from build123d import *

# Parameters (mm, degrees)
SKETCH001_W  = 7
SKETCH001_H  = 7
PAD001_DEPTH = 2
SKETCH_R     = 2.5
PAD_DEPTH    = 100


with BuildPart() as pad001:
    # Sketch001 → Pad001 (new body)
    with BuildSketch(Plane.YZ.offset(2)):
        with Locations((0, 59.5)):
            Rectangle(SKETCH001_W, SKETCH001_H)
    extrude(amount=PAD001_DEPTH)


with BuildPart() as cut:
    # Sketch → Pad (new body)
    with BuildSketch(Plane.XY):
        Circle(SKETCH_R)
    extrude(amount=PAD_DEPTH)

    # Cut: cut Pad001
    add(pad001.part, mode=Mode.SUBTRACT)


solid = cut.part
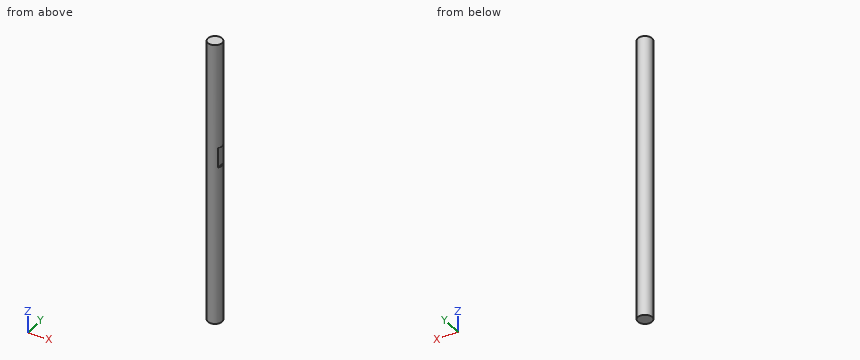
The model under review builds one solid part; all positions refer to its coordinate system, in mm. Coordinates: 2 decimals unless noted, no trailing zeros. Order: outer loops, then holes, each group sorted by start corner. A loop starts at its lowest first (then second) coordinate and runs counter-clockwise, first axis right, second up. Notation, with made-up numbers: (14.5, -13.75) -> (62.5, -13.75) arc R15 cw to (62.5, 3.25) -> close; hole circle Ø11 at (71, 89.5). An arc over 180 degrees is marked (long way). Answer in a Markdown table with one row per item.
(1) Consider section B-B (x = -1.5). Write out the cut boundary in (y, z), plus the area to 3 significant figures.
Answers:
| item | result |
|---|---|
| outline | (-2, 0) -> (2, 0) -> (2, 100) -> (-2, 100) -> close |
| area | 400 mm² |
(2) Insertion check: pin 1 (2 mm diameter, centred on y = 1, z = 60, fed in from -X); pin 2 (0.9 mm diameter, centred on y = -0.5, z = 58.5, fed in from +X). Each pin has a flat end and moves straight along its axis. Give the tip position at first contact, or say it passes through.
Answers:
| item | result |
|---|---|
| pin 1 | x = -2.5 |
| pin 2 | x = 2 |
(3) Wall thickness on line 1 along Y through (x, z) = (0.25, 24); line 2 along X through (y, z) = (0.85, 44): over which ranges is each line inside the solid? List them lowest first.
Answers:
| item | result |
|---|---|
| line 1 | -2.49 to 2.49 |
| line 2 | -2.35 to 2.35 |
(4) Consider section A-A (z = 89). Write out the cut boundary in (x, y), plus the area to 3 significant figures.
Answers:
| item | result |
|---|---|
| outline | circle Ø5 at (0, 0) |
| area | 19.6 mm² |
